Check sheet for the drawn part. Datum: minimum x, y, z corner. Units: mm. A direction names the side the tool comes from. Round coordinates to 2 decimals unless told otherwise and drop trailing zeros. Write each loop counter-clockwise with the first axis right and the second up, starting at its lowest first coordinate (ties: lowest second). Pieces come first, ordered by that corner, then holes. Notation, with made-up numbers: (46, -4) -> (93, -4) arc R13 cw to (93, 0) -> close; hole circle Ø1 at (-12.5, -14). An arc over 180 degrees is marked (long way). Use a Markdown table: item, result.
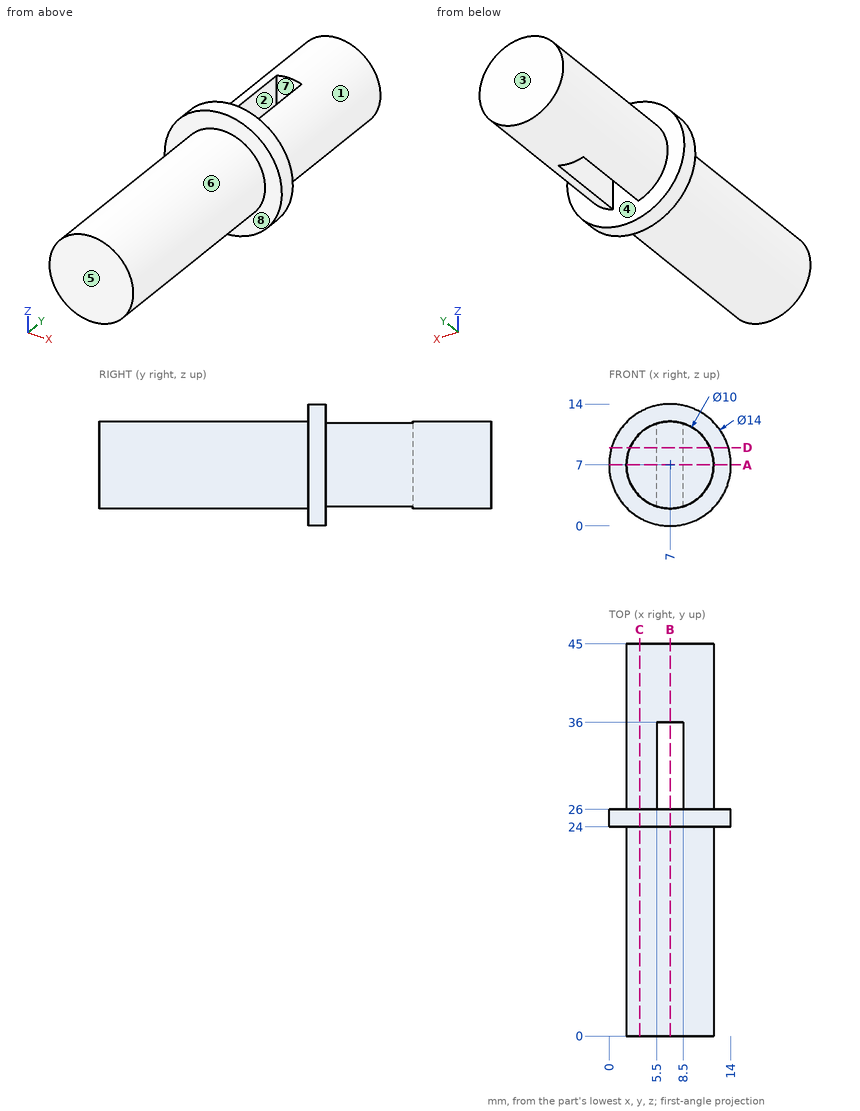
(1) Section check C-C on x = 3.5. Record the cut outline in (y, z).
A:
| item | result |
|---|---|
| outline | (0, 3.43) -> (24, 3.43) -> (24, 0.94) -> (26, 0.94) -> (26, 3.43) -> (45, 3.43) -> (45, 10.57) -> (26, 10.57) -> (26, 13.06) -> (24, 13.06) -> (24, 10.57) -> (0, 10.57) -> close |
(2) Section check D-D on z = 9. Record the cut outline in (x, y).
A:
| item | result |
|---|---|
| outline | (0.29, 24) -> (2.42, 24) -> (2.42, 0) -> (11.58, 0) -> (11.58, 24) -> (13.71, 24) -> (13.71, 26) -> (11.58, 26) -> (11.58, 45) -> (2.42, 45) -> (2.42, 26) -> (0.29, 26) -> close; hole (5.5, 26) -> (8.5, 26) -> (8.5, 36) -> (5.5, 36) -> close |
(3) Section check B-B on x = 7. Record the cut outline in (y, z), plus the area to 3 significant figures.
A:
| item | result |
|---|---|
| outline | (0, 2) -> (24, 2) -> (24, 0) -> (26, 0) -> (26, 14) -> (24, 14) -> (24, 12) -> (0, 12) -> close; (36, 2) -> (45, 2) -> (45, 12) -> (36, 12) -> close |
| area | 358 mm2 |
(4) Access from +Z, -Z, +X, -X, +Y, -Y to the whole of each face (thin tool, end or side, straight path). Record for the marked faces 1, 2, 3, 4 and 5.
A:
| item | result |
|---|---|
| face 1 | +Y |
| face 2 | +Z, -Z |
| face 3 | +Z, -Z, +X, -X, +Y |
| face 4 | none |
| face 5 | +Z, -Z, +X, -X, -Y |
(5) Release check for a two-part mould opening along Y. For the marked faces 6, 7 and 8 record: +Y half, -Y half, draft (parallel to the pull), parting line (faces both ways), or undercut.
A:
| item | result |
|---|---|
| face 6 | draft |
| face 7 | undercut |
| face 8 | -Y half |
(6) Section check A-A on z = 7. Record the cut outline in (x, y).
A:
| item | result |
|---|---|
| outline | (0, 24) -> (2, 24) -> (2, 0) -> (12, 0) -> (12, 24) -> (14, 24) -> (14, 26) -> (12, 26) -> (12, 45) -> (2, 45) -> (2, 26) -> (0, 26) -> close; hole (5.5, 26) -> (8.5, 26) -> (8.5, 36) -> (5.5, 36) -> close |
(7) Thickness scan on line 1 (Y direction, x = 5.75, z = 6.5); line 2 (Y direction, x = 10.5, z = 12.5); line 3 (Z direction, x = 6.75, y = 42). Record the ranges inside material, lowest first.
A:
| item | result |
|---|---|
| line 1 | y = 0 to 26, 36 to 45 |
| line 2 | y = 24 to 26 |
| line 3 | z = 2.01 to 11.99 |
(8) Gauge pin test, flat ends, axial feed: pin 1 Ø8 at (x, y) = (7.5, 5.5) entering from -Z; pin 2 Ø3 at (y, z) = (33, 2.5) entering from +X; pin 3 Ø3 at (y, z) = (6.5, 11.5) entering from -X. Record the tip position at first contact, or that the pin passes through.
A:
| item | result |
|---|---|
| pin 1 | stops at z = 2 |
| pin 2 | stops at x = 11 |
| pin 3 | stops at x = 3 |
